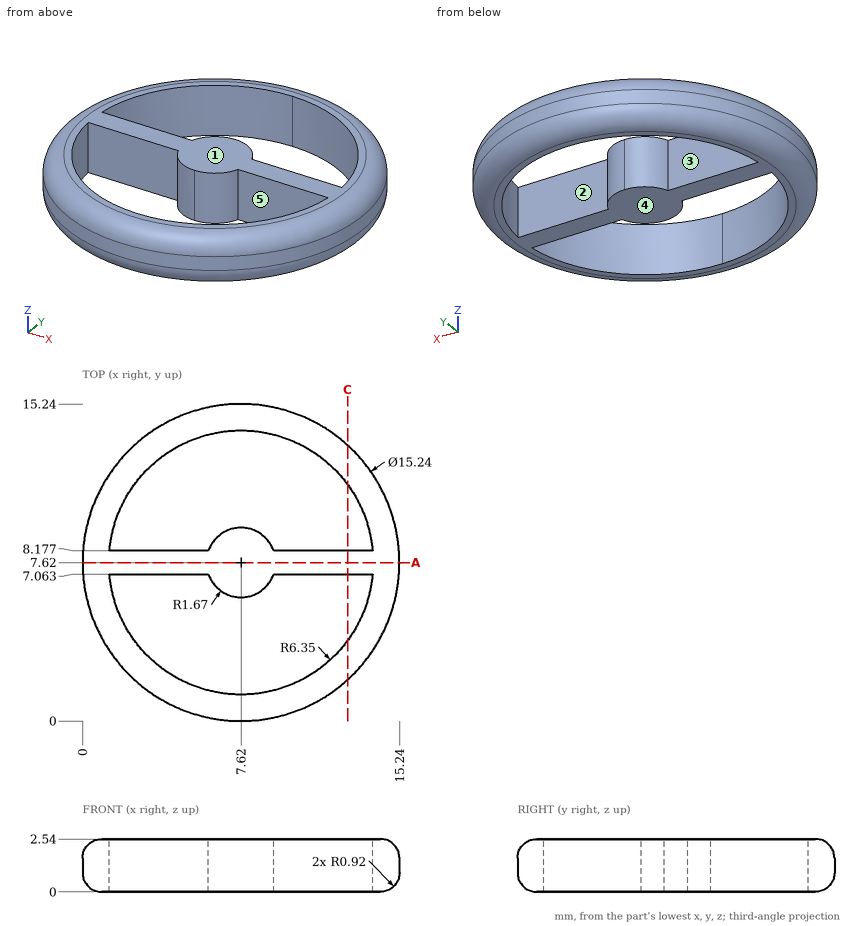
Answer from the drawing. Dimensions are ordinates in mm from the lowest x, y and z of the part. A direction names the side the tool comes from. Coordinates: 2 decimals unless noted, no trailing zeros. Order: outer loops, then holes, each group sorted by start corner. A loop starts at its lowest first (then second) coordinate and runs counter-clockwise, first axis right, second up. Notation, with made-up numbers: (24.25, 88) -> (35.25, 88) arc R25 cw to (35.25, 114) -> close; hole circle Ø10 at (-35, 77.25). An arc over 180 degrees is marked (long way). Answer as a JSON object with one key per item and string values.
1) A cutting plane is placed at C-C, the plane x = 12.75. State how many separate pieces and enclosed holes the cut face has, plus the area to 3 significant figures.
Model answer:
{"separate pieces": "3", "enclosed holes": "0", "area": "11.4 mm²"}
2) A cutting plane is placed at A-A, the plane y = 7.62. Determine the outline of the cut face in (x, z), plus the area to 3 significant figures.
Model answer:
{"outline": "(0, 0.92) arc R0.92 ccw to (0.92, 0) -> (14.32, 0) arc R0.92 ccw to (15.24, 0.92) -> (15.24, 1.62) arc R0.92 ccw to (14.32, 2.54) -> (0.92, 2.54) arc R0.92 ccw to (0, 1.62) -> close", "area": "38.0 mm²"}
3) Each of these flat-tipped pins is pushed along its axis until it touches: pin 1 (1.3 mm diameter, centred on x = 11, z = 1, fed in from -Y); pin 2 (1 mm diameter, centred on x = 6, z = 1, fed in from +Y). Where does it stop, or does it pass through?
Model answer:
{"pin 1": "stops at y = 0.51", "pin 2": "stops at y = 15.16"}
4) A tool of negligible diameter and unlimited length cuts with its end or side. For the marked faces 4 and 5, from which of +Z, -Z, +X, -X, +Y, -Y can it reach the whole face along a straight path? Write none if from no direction.
Model answer:
{"face 4": "-Z, +X, -X, +Y, -Y", "face 5": "+Z, -Z"}
5) Consider line 1 along Y through (x, z) = (5, 0.65) (1 decimal); line 2 along X through (y, z) = (8.25, 1.6); line 3 along Y through (x, z) = (10.75, 2.3) (1 decimal). Determine where each line is inside the solid, lowest interval first. Write a range as from..to.
Model answer:
{"line 1": "y = 0.5..1.8, 7.1..8.2, 13.4..14.7", "line 2": "x = 0.03..1.3, 6.07..9.17, 13.94..15.21", "line 3": "y = 1..2.1, 7.1..8.2, 13.1..14.2"}
6) The mould has two halves that part along X. Classify the marked faces 1, 2 and 3: released by +X, released by -X, zero draft, split by the parting line, or undercut.
Model answer:
{"face 1": "zero draft", "face 2": "undercut", "face 3": "undercut"}
